Autodesk Inventor part; units mm, degrees
ref_plane "YZ Plane" through (0, 0, 0) normal (1, 0, 0) x (0, 1, 0)
ref_plane "XZ Plane" through (0, 0, 0) normal (0, 1, 0) x (-1, 0, 0)
ref_plane "XY Plane" through (0, 0, 0) normal (0, 0, 1) x (1, 0, 0)
sketch "スケッチ1" plane through (0, 0, 0) normal (0, 0, 1) x (1, 0, 0)
  circle A0 centre (-3.9908, -3.6656) radius 1
  circle A1 centre (-24.9908, -24.6656) radius 1
  line L0 (-3.9908, -3.6656) -> (-24.9908, -3.6656) construction
  line L1 (-24.9908, -3.6656) -> (-24.9908, -24.6656) construction
  line L2 (-24.9908, -24.6656) -> (-3.9908, -24.6656) construction
  line L3 (-3.9908, -24.6656) -> (-3.9908, -3.6656) construction
  circle A2 centre (-3.9908, -3.6656) radius 1.1
  circle A3 centre (-24.9908, -3.6656) radius 1.1
  circle A4 centre (-3.9908, -24.6656) radius 1.1
  circle A5 centre (-24.9908, -24.6656) radius 1.1
  circle A6 centre (-24.9908, -14.1656) radius 8
  circle A7 centre (-24.9908, -24.6656) radius 2
  circle A8 centre (-3.9908, -24.6656) radius 2
  circle A9 centre (-24.9908, -3.6656) radius 2
  circle A10 centre (-3.9908, -3.6656) radius 2
  line L4 (-24.9908, -26.6656) -> (-1.9908, -26.6656)
  line L5 (-3.9908, -26.6656) -> (-3.9908, -22.6656)
  line L6 (-3.9908, -22.6656) -> (-24.9908, -22.6656)
  line L7 (-24.9908, -22.6656) -> (-24.9908, -26.6656)
  line L8 (-5.9908, -24.6656) -> (-1.9908, -24.6656)
  line L9 (-1.9908, -24.6656) -> (-1.9908, -3.6656)
  line L10 (-1.9908, -3.6656) -> (-5.9908, -3.6656)
  line L11 (-5.9908, -3.6656) -> (-5.9908, -24.6656)
  line L12 (18.0092, -24.1656) -> (8.0092, -24.1656)
  line L13 (8.0092, -24.1656) -> (8.0092, -21.1656)
  line L14 (8.0092, -21.1656) -> (18.0092, -21.1656)
  line L15 (18.0092, -21.1656) -> (18.0092, -24.1656)
  line L16 (38.0092, -24.1656) -> (28.0092, -24.1656)
  line L17 (28.0092, -24.1656) -> (28.0092, -21.1656)
  line L18 (28.0092, -21.1656) -> (38.0092, -21.1656)
  line L19 (38.0092, -21.1656) -> (38.0092, -24.1656)
  circle A11 centre (16.9092, -24.1656) radius 1.1
  line L20 (13.0092, -24.1656) -> (13.0092, -21.1656) construction
  line L21 (13.0092, -22.6656) -> (18.0092, -22.6656) construction
  line L22 (28.0092, -22.6656) -> (18.0092, -22.6656) construction
  line L23 (23.0092, -22.6656) -> (23.0092, -26.0364) construction
  circle A12 centre (9.1092, -24.1656) radius 1.1
  circle A13 centre (16.9092, -21.1656) radius 1.1
  circle A14 centre (9.1092, -21.1656) radius 1.1
  circle A15 centre (29.1092, -24.1656) radius 1.1
  circle A16 centre (36.9092, -24.1656) radius 1.1
  circle A17 centre (29.1092, -21.1656) radius 1.1
  circle A18 centre (36.9092, -21.1656) radius 1.1
  line L24 (42.0092, -26.6656) -> (-1.9908, -26.6656)
  line L25 (-1.9908, -26.6656) -> (-1.9908, -18.1656)
  line L26 (-1.9908, -18.1656) -> (42.0092, -18.1656)
  line L27 (42.0092, -18.1656) -> (42.0092, -26.6656)
  circle A19 centre (38.0092, -22.6656) radius 4
  arc A20 (-2.5997, -2.2287) -> (38.0092, -18.6656) centre (38.0092, 39.7168) ccw
  circle A21 centre (23.0092, -22.6656) radius 1.1
  circle A22 centre (3.0092, -22.6656) radius 1.1
  line L28 (38.0092, -18.6656) -> (-1.9908, -18.6656) construction
  point P0 (0, 0)
  point P1 (38.0092, -26.6656)
  point P2 (-5.9908, -22.6656)
  point P3 (15.8092, -24.1656)
  point P4 (10.2092, -24.1656)
  point P5 (10.2092, -21.1656)
  point P6 (15.8092, -21.1656)
  point P7 (35.8092, -21.1656)
  point P8 (35.8092, -24.1656)
  point P9 (30.2092, -24.1656)
  point P10 (30.2092, -21.1656)
  point P11 (30.3847, -18.1656)
  point P12 (42.0092, -22.6656)
  dimension "d11" = 4
  dimension "d24" = 2.2
  dimension "d0" = 21
  dimension "d1" = 21
  dimension "d2" = 2.2
  dimension "d5" = 21
  dimension "d8" = 21
  dimension "d14" = 21
  dimension "d17" = 21
  dimension "d20" = 10
  dimension "d21" = 3
  dimension "d22" = 10
  dimension "d23" = 3
  dimension "d25" = 2.5
  dimension "d26" = 3
  dimension "d28" = 10
  dimension "d29" = 10
  dimension "d31" = 2.2
extrude "押し出し1" add sketch "スケッチ1" along normal blind 1.5 contours L10 A10 A2 | A2 L10 A10 | L9 A8 L6 L11 A10 | A10 A20 L26 L9 | L26 A20 A19 L18 A17 L17 A15 L16 L24 L25 L9 | L11 A8 L4 A7 L6 | L6 A8 L11 | L8 A4 L5 A8 | L25 L4 A8 | A8 L5 A4 L8 | L5 A4 L8 A8 | L7 A5 A7 | A7 L7 A5 | L8 A4 L5 A8 | A19 L16 A16 L19 A18 L18 picked at (39.3425, -22.6656)
fillet "フィレット1" radius 2 1 edges at (-5.9908, -22.6656, 0.75)
sketch "スケッチ2" plane through (0, 0, 1.5) normal (0, 0, 1) x (1, 0, 0)
  line L0 (-24.9908, -26.6656) -> (38.0092, -26.6656)
  arc A0 (38.0092, -26.6656) -> (38.0092, -18.6656) centre (38.0092, -22.6656) ccw
  arc A1 (-2.5997, -2.2287) -> (38.0092, -18.6656) centre (38.0092, 39.7168) ccw
  arc A2 (-2.5997, -2.2287) -> (-5.9908, -3.6656) centre (-3.9908, -3.6656) ccw
  line L1 (-5.9908, -3.6656) -> (-5.9908, -20.6656)
  arc A3 (-7.9908, -22.6656) -> (-5.9908, -20.6656) centre (-7.9908, -20.6656) ccw
  line L2 (-7.9908, -22.6656) -> (-24.9908, -22.6656)
  arc A4 (-24.9908, -22.6656) -> (-24.9908, -26.6656) centre (-24.9908, -24.6656) ccw
  circle A5 centre (-24.9908, -24.6656) radius 1.1
  circle A6 centre (-3.9908, -3.6656) radius 1.1
  circle A7 centre (-3.9908, -24.6656) radius 1.1
  line L3 (18.0092, -21.1656) -> (18.0092, -24.1656)
  arc A8 (15.8092, -24.1656) -> (18.0092, -24.1656) centre (16.9092, -24.1656) ccw
  line L4 (15.8092, -24.1656) -> (10.2092, -24.1656)
  arc A9 (8.0092, -24.1656) -> (10.2092, -24.1656) centre (9.1092, -24.1656) ccw
  line L5 (8.0092, -24.1656) -> (8.0092, -21.1656)
  arc A10 (10.2092, -21.1656) -> (8.0092, -21.1656) centre (9.1092, -21.1656) ccw
  line L6 (10.2092, -21.1656) -> (15.8092, -21.1656)
  arc A11 (18.0092, -21.1656) -> (15.8092, -21.1656) centre (16.9092, -21.1656) ccw
  circle A12 centre (3.0092, -22.6656) radius 1.1
  circle A13 centre (23.0092, -22.6656) radius 1.1
  line L7 (30.2092, -21.1656) -> (35.8092, -21.1656)
  arc A14 (38.0092, -21.1656) -> (35.8092, -21.1656) centre (36.9092, -21.1656) ccw
  line L8 (38.0092, -21.1656) -> (38.0092, -24.1656)
  arc A15 (35.8092, -24.1656) -> (38.0092, -24.1656) centre (36.9092, -24.1656) ccw
  line L9 (35.8092, -24.1656) -> (30.2092, -24.1656)
  arc A16 (28.0092, -24.1656) -> (30.2092, -24.1656) centre (29.1092, -24.1656) ccw
  line L10 (28.0092, -24.1656) -> (28.0092, -21.1656)
  arc A17 (30.2092, -21.1656) -> (28.0092, -21.1656) centre (29.1092, -21.1656) ccw
  line L11 (38.0092, -24.6656) -> (-7.9908, -24.6656)
  arc A18 (-7.9908, -24.6656) -> (-3.9908, -20.6656) centre (-7.9908, -20.6656) ccw
  line L12 (-3.9908, -16.0656) -> (-3.9908, -8.1535)
  arc A19 (-0.7084, -6.6187) -> (38.0092, -20.6656) centre (38.0092, 39.7168) ccw
  arc A20 (38.0092, -24.6656) -> (38.0092, -20.6656) centre (38.0092, -22.6656) ccw
  arc A21 (-0.7084, -6.6187) -> (-3.9908, -8.1535) centre (-1.9908, -8.1535) ccw
  line L13 (20.4813, -18.0656) -> (-1.9908, -18.0656)
  arc A22 (-3.9908, -16.0656) -> (-1.9908, -18.0656) centre (-1.9908, -16.0656) ccw
  point P0 (0, 0)
  point P1 (-3.9908, -3.6656)
  point P2 (17.4157, -17.0454)
  point P3 (-3.9908, -15.0454)
  point P4 (9.1092, -20.0656)
  point P5 (9.2452, -18.0656)
  dimension "d35" = 2
  dimension "d36" = 2
  dimension "d40" = 2
  dimension "d41" = 2
extrude "押し出し2" cut sketch "スケッチ2" against normal blind 1.5 contours L13 A22 L12 A21 A19
fillet "フィレット2" [suppressed]
fillet "フィレット3" radius 2 1 edges at (20.4813, -18.0656, 0.75)
equation "\"d5\" = d0"
equation "\"d8\" = d1"
properties part number "3304_tesaki" material "アルミニウム 2014-T4"
The listing builds one solid part. Answer for the finished solid, in the listing's coordinates (mm). A direction names the side the tool comes from. Coordinates: 2 decimals unless noted, no trailing zeros. Loops run counter-clockwise (first coordinate to the right, second up) from the corner with the lowest first, then second, coordinate; pieces in that order, holes last. Notation, with made-up numbers: (-10.5, -7) -> (5.5, -7) arc R19 ccw to (5.5, 0) -> close; hole circle Ø3 at (-31.5, -10). An arc over 180 degrees is marked (long way). Answer in a Markdown table with one row per item. Add a question column.
1. The part is cut by section B-B, the plane x = 25. Write down the section's boundary in (y, z), then the cut area to 3 significant figures.
2. The part is cut by section C-C, the plane x = -23. Write down the section's boundary in (y, z).
3. Consider line 1 (X direction, y = -9, z = 0.9); line 2 (Y direction, x = 23, z = 1.45); line 3 (Y direction, x = 10.5, z = 1.25). Determine where each line is inside the solid, lowest interval first. Write a range as [from, to].
4. The part is cut by section A-A, the plane z = 0.4. Count the separate pieces of the cut face and the enclosed holes in it, then the cut area to 3 significant figures.
5. A flat-ended cylindrical pin translates along its axis: P1, Ø0.8, axis at y = -22.5, z = 0.5, coming from the -X side. Find the tip coordinate at first contact, or state that the pin passes through.
6. Determine the mould class of faces 1 (the cylindrical face through (-25.8, -25.41, 0.74)), 2 (the flat face through (10, -19, 0)), 3 (the cylindrical face through (-6.592, -22.095, 0.76)), 4 (the cylindrical face through (42.01, -22.58, 0.74)) for opening direction Y: +Y half, -Y half, draft (parallel to the pull), parting line (faces both ways), or undercut.
7. For faces 5 (the cylindrical face through (29.085, -20.066, 0.74)), 6 (the flat face through (-16, -22.666, 1)), determine the directions among +Z, -Z, +X, -X, +Y, -Y from which every point of the face is accessible in a straight line to the end or side of a thin tool.
Answer below:
| question | item | result |
|---|---|---|
| 1 | outline | (-26.67, 0) -> (-17.2, 0) -> (-17.2, 1.5) -> (-26.67, 1.5) -> close |
| 1 | area | 14.2 mm2 |
| 2 | outline | (-26.67, 0) -> (-22.67, 0) -> (-22.67, 1.5) -> (-26.67, 1.5) -> close |
| 3 | line 1 | [-5.99, -3.99], [2.33, 5.83] |
| 3 | line 2 | [-26.67, -23.77], [-21.57, -16.7] |
| 3 | line 3 | [-26.67, -24.17], [-21.17, -18.02], [-14.04, -11.78] |
| 4 | separate pieces | 1 |
| 4 | enclosed holes | 8 |
| 4 | area | 506 mm2 |
| 5 | P1 | x = -25.93 |
| 6 | face 1 | undercut |
| 6 | face 2 | draft |
| 6 | face 3 | +Y half |
| 6 | face 4 | parting line |
| 7 | face 5 | +Z, -Z |
| 7 | face 6 | +Z, -Z, -X, +Y |
